Could you check a few things on this model? Use its own coordinates, in mm. A direction names the side the tool comes from. Give positions to 0.01 mm unless a question says otherwise; leave off trailing zeros. Put each result on its own line as item: value.
from build123d import *

# Parameters (mm, degrees)
SKETCH1_R           = 175
BOSS_EXTRUDE1_DEPTH = 4.75
CUT_EXTRUDE1_DEPTH  = 4.75
SKETCH4_R           = 2
CUT_EXTRUDE2_DEPTH  = 248.532952352
SKETCH5_R           = 1.5
CUT_EXTRUDE3_DEPTH  = 248.532952352


with BuildPart() as part:
    # Sketch1 → Boss-Extrude1 (new body)
    with BuildSketch(Plane(origin=(0, 0, 0), x_dir=(1, 0, 0), z_dir=(0, 1, 0))):
        with Locations(Location((0, 0, 0), (0, 0, 270))):
            Circle(SKETCH1_R)
    extrude(amount=BOSS_EXTRUDE1_DEPTH)

    # Sketch2 → Cut-Extrude1 (cut)
    with BuildSketch(Plane(origin=(0, 4.75, 0), x_dir=(1, 0, 0), z_dir=(0, 1, 0))):
        Polygon((33.00597779, -123.564301803), (23.964219805, -119.29269642), (21.935207248, -123.587531462), (30.976965232, -127.859136846), align=None)
        Polygon((-13.785119779, -101.458743944), (-22.826877764, -97.18713856), (-24.855890321, -101.481973603), (-15.814132337, -105.753578986), align=None)
        Polygon((-107.367314918, -57.247628225), (-116.409072902, -52.976022841), (-118.438085459, -57.270857884), (-109.396327475, -61.542463267), align=None)
        Polygon((-101.458743944, 13.785119779), (-97.18713856, 22.826877764), (-101.481973603, 24.855890321), (-105.753578986, 15.814132337), align=None)
        Polygon((-123.564301803, -33.00597779), (-119.29269642, -23.964219805), (-123.587531462, -21.935207248), (-127.859136846, -30.976965232), align=None)
        Polygon((107.367314918, 57.247628225), (116.409072902, 52.976022841), (118.438085459, 57.270857884), (109.396327475, 61.542463267), align=None)
        Polygon((-57.247628225, 107.367314918), (-52.976022841, 116.409072902), (-57.270857884, 118.438085459), (-61.542463267, 109.396327475), align=None)
        Polygon((60.576217349, 79.353186084), (69.617975333, 75.081580701), (71.64698789, 79.376415743), (62.605229906, 83.648021127), align=None)
        Polygon((13.785119779, 101.458743944), (22.826877764, 97.18713856), (24.855890321, 101.481973603), (15.814132337, 105.753578986), align=None)
        Polygon((-33.00597779, 123.564301803), (-23.964219805, 119.29269642), (-21.935207248, 123.587531462), (-30.976965232, 127.859136846), align=None)
        Polygon((-79.353186084, 60.576217349), (-75.081580701, 69.617975333), (-79.376415743, 71.64698789), (-83.648021127, 62.605229906), align=None)
        Polygon((-60.576217349, -79.353186084), (-69.617975333, -75.081580701), (-71.64698789, -79.376415743), (-62.605229906, -83.648021127), align=None)
        Polygon((123.564301803, 33.00597779), (119.29269642, 23.964219805), (123.587531462, 21.935207248), (127.859136846, 30.976965232), align=None)
        Polygon((101.458743944, -13.785119779), (97.18713856, -22.826877764), (101.481973603, -24.855890321), (105.753578986, -15.814132337), align=None)
        Polygon((79.353186084, -60.576217349), (75.081580701, -69.617975333), (79.376415743, -71.64698789), (83.648021127, -62.605229906), align=None)
        Polygon((57.247628225, -107.367314918), (52.976022841, -116.409072902), (57.270857884, -118.438085459), (61.542463267, -109.396327475), align=None)
    extrude(amount=-CUT_EXTRUDE1_DEPTH, mode=Mode.SUBTRACT)

    # Sketch4 → Cut-Extrude2 (cut, through all)
    with BuildSketch(Plane(origin=(0, 4.75, 0), x_dir=(1, 0, 0), z_dir=(0, 1, 0))):
        with Locations(Location((-77.507691728, -127.482700681, 0), (0, 0, 270))):
            Circle(SKETCH4_R)
        with Locations(Location((-37.567601624, -113.172242879, 0), (0, 0, 270))):
            Circle(SKETCH4_R)
        Polygon((-47.128974969, -121.705714608), (-65.212490938, -113.162503842), (-67.946318383, -118.949228952), (-49.862802415, -127.492439718), align=None)
    extrude(amount=-CUT_EXTRUDE2_DEPTH, mode=Mode.SUBTRACT)

    # Sketch5 → Cut-Extrude3 (cut, through all)
    with BuildSketch(Plane(origin=(0, 4.75, 0), x_dir=(1, 0, 0), z_dir=(0, 1, 0))):
        with Locations(Location((42.716053835, 90.417579844, 0), (0, 0, 270))):
            Circle(SKETCH5_R)
        with Locations(Location((90.417579844, -42.716053835, 0), (0, 0, 270))):
            Circle(SKETCH5_R)
        with Locations(Location((-42.716053835, -90.417579844, 0), (0, 0, 270))):
            Circle(SKETCH5_R)
        with Locations(Location((-90.417579844, 42.716053835, 0), (0, 0, 270))):
            Circle(SKETCH5_R)
    extrude(amount=-CUT_EXTRUDE3_DEPTH, mode=Mode.SUBTRACT)


solid = part.part
1) We'd pull the mould along Z, two halves only. Please class faces 3 (the flat face through (2, 0, -2)), 4 (the flat face through (-59.03, 2.41, 123.16)), 5 (the cylindrical face through (173.51, 2.34, -22.78)): pulls with the +Z half, pulls with the -Z half, needs draft (parallel to the pull), parting line crosses it, or undercut.
Filled in:
face 3: needs draft
face 4: undercut
face 5: parting line crosses it
2) Suppose I cut it at A-A, the plane y = 0.95. State how many separate pieces and enclosed holes the cut face has, and give its area (3 significant figures).
Filled in:
separate pieces: 1
enclosed holes: 23
area: 95,300 mm^2
3) I'm going to push flat-ended pins straight in: pin 1 (2 mm diameter, centred on y = 2.5, z = -80, fed in from +X); pin 2 (1.5 mm diameter, centred on y = 3.5, z = 8.5, fed in from -X); pin 3 (2 mm diameter, centred on x = -123.5, y = 2, fed in from +Z) (3 decimals). Where does each tip first touch, or does it pass through?
Filled in:
pin 1: stops at x = 156.15
pin 2: stops at x = -174.83
pin 3: stops at z = 124.975
4) Which directions (+Z, -Z, +X, -X, +Y, -Y) give clear straight access to the entire face, cutting with the end or side of a thin tool? Please do faces 1 (the flat face through (-56.044, 2.408, 117.494)), 2 (the flat face through (2, 4.75, -2)).
Filled in:
face 1: +Y, -Y
face 2: +Z, -Z, +X, -X, +Y
5) If I drill on line 1 (X direction, y = 3.65, z = 117); line 2 (X direction, y = 4.2, z = -32); line 3 (Z direction, x = 81, y = 2.55), over which ranges is the centre line in solid material (lowest first)? Write a range as [from, to].
Filled in:
line 1: x = [-130.14, -67.03], [-57.09, 54.23], [57.95, 130.14]
line 2: x = [-172.05, 123.09], [125.69, 172.05]
line 3: z = [-155.13, 61.35], [68.21, 155.13]
